```python
from build123d import *

# Parameters (mm, degrees)
BOSS_EXTRUDE1_DEPTH = 11.938
CUT_EXTRUDE1_DEPTH  = 11.43
SKETCH3_W           = 27.94
SKETCH3_H           = 25.845942769
CUT_EXTRUDE2_DEPTH  = 10.668
SKETCH4_R           = 1.905
CUT_EXTRUDE3_DEPTH  = 8.636
SKETCH5_R           = 1.143
CUT_EXTRUDE4_DEPTH  = 21.59
CUT_EXTRUDE5_DEPTH  = 2.54


with BuildPart() as part:
    # Sketch1 → Boss-Extrude1 (new body)
    with BuildSketch(Plane.XY):
        with BuildLine():
            Line((-4.737825132, -30.035944056), (-14.890307558, -23.641538462))
            ThreePointArc((-14.890307558, -23.641538462), (-27.242520167, -6.203925768), (-23.658870968, 14.862752926))
            ThreePointArc((-23.658870968, 14.862752926), (-20.55370118, 20.591203739), (-18.20732863, 26.67))
            Line((-18.20732863, 26.67), (18.20732863, 26.67))
            ThreePointArc((18.20732863, 26.67), (20.55370118, 20.591203739), (23.658870968, 14.862752926))
            ThreePointArc((23.658870968, 14.862752926), (27.242520167, -6.203925768), (14.890307558, -23.641538462))
            Line((14.890307558, -23.641538462), (4.737825132, -30.035944056))
            ThreePointArc((4.737825132, -30.035944056), (0, -31.403636364), (-4.737825132, -30.035944056))
        make_face()
    extrude(amount=BOSS_EXTRUDE1_DEPTH)

    # Sketch2 → Cut-Extrude1 (cut)
    with BuildSketch(Plane(origin=(0, 0, 0), x_dir=(-1, 0, 0), z_dir=(0, 0, -1))):
        with BuildLine():
            Line((-11.733590414, 23.241), (11.733590414, 23.241))
            ThreePointArc((11.733590414, 23.241), (0, -26.035), (-11.733590414, 23.241))
        make_face()
    extrude(amount=-CUT_EXTRUDE1_DEPTH, mode=Mode.SUBTRACT)

    # Sketch3 → Cut-Extrude2 (cut)
    with BuildSketch(Plane(origin=(0, 0, 0), x_dir=(-1, 0, 0), z_dir=(0, 0, -1))):
        with Locations((0, 24.280777857)):
            Rectangle(SKETCH3_W, SKETCH3_H)
    extrude(amount=-CUT_EXTRUDE2_DEPTH, mode=Mode.SUBTRACT)

    # Sketch4 → Cut-Extrude3 (cut)
    with BuildSketch(Plane.XY.offset(11.938)):
        with Locations((0, -28.575)):
            Circle(SKETCH4_R)
        with Locations((-16.764, 23.241)):
            Circle(SKETCH4_R)
        with Locations((16.764, 23.241)):
            Circle(SKETCH4_R)
    extrude(amount=-CUT_EXTRUDE3_DEPTH, mode=Mode.SUBTRACT)

    # Sketch5 → Cut-Extrude4 (cut)
    with BuildSketch(Plane.XY.offset(3.302)):
        with Locations((-16.764, 23.241)):
            Circle(SKETCH5_R)
        with Locations((16.764, 23.241)):
            Circle(SKETCH5_R)
        with Locations((0, -28.575)):
            Circle(SKETCH5_R)
    extrude(amount=-CUT_EXTRUDE4_DEPTH, mode=Mode.SUBTRACT)

    # Sketch6 → Cut-Extrude5 (cut)
    with BuildSketch(Plane(origin=(0, 0, 0), x_dir=(-1, 0, 0), z_dir=(0, 0, -1))):
        with BuildLine():
            Line((-23.658870968, 14.862752926), (-4.737825132, -30.035944056))
            ThreePointArc((-4.737825132, -30.035944056), (0, -31.403636364), (4.737825132, -30.035944056))
            Line((4.737825132, -30.035944056), (23.658870968, 14.862752926))
            ThreePointArc((23.658870968, 14.862752926), (20.55370118, 20.591203739), (18.20732863, 26.67))
            Line((18.20732863, 26.67), (-18.20732863, 26.67))
            ThreePointArc((-18.20732863, 26.67), (-20.55370118, 20.591203739), (-23.658870968, 14.862752926))
        make_face()
    extrude(amount=-CUT_EXTRUDE5_DEPTH, mode=Mode.SUBTRACT)


solid = part.part
```
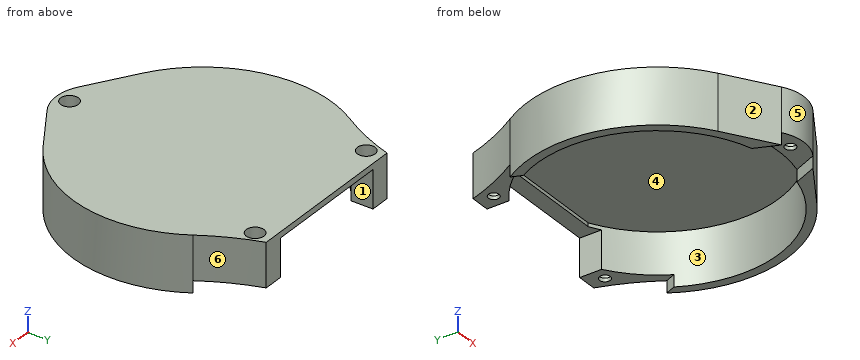
Geometry check sheet. Reference: the model listing, model coordinates, mm. Face numbers are marked on the shaded views. A direction names the side the tool comes from. Coordinates: 2 decimals unless noted, no trailing zeros. Write each loop counter-clockwise with the first axis right and the second up, starting at its lowest first coordinate (ties: lowest second). Pieces come first, ordered by that corner, then holes. Notation, with made-up numbers: M 10.25,9 L 56.25,9 A23 cw 56.25,40 Z; hole C 23,87.25 d9. An arc over 180 degrees is marked long. Answer as a JSON object with one key per item and string values.
1. Section check C-C, the plane y = 0. Enter the section's corners in (x, z) (3 decimals).
Answers below:
{"outline": "M -27.94,0 L -26.035,0 L -26.035,11.43 L 26.035,11.43 L 26.035,0 L 27.94,0 L 27.94,11.938 L -27.94,11.938 Z"}
2. Section check A-A, the plane z = 1.25. Enter the section's corners in (x, y) (3 decimals).
Answers below:
{"outline": "M -23.659,14.863 A27.94 ccw -14.89,-23.642 L -4.738,-30.036 L -6.805,-25.13 A26.035 cw -22.739,12.679 Z; M 4.738,-30.036 L 14.89,-23.642 A27.94 ccw 23.659,14.863 L 22.739,12.679 A26.035 cw 6.805,-25.13 Z"}
3. Section check B-B, the plane x = 0. Enter the section's corners in (y, z) (3 decimals).
Answers below:
{"outline": "M -31.404,2.54 L -29.718,2.54 L -29.718,3.302 L -30.48,3.302 L -30.48,11.938 L -31.404,11.938 Z; M -27.432,2.54 L -26.035,2.54 L -26.035,11.43 L 23.241,11.43 L 23.241,10.668 L 26.67,10.668 L 26.67,11.938 L -26.67,11.938 L -26.67,3.302 L -27.432,3.302 Z"}
4. Draft check along Y on the marked faces 3, 4, 5 and 6. Enter one of: released by +Y, released by -Y, zero draft, split by the parting line, or undercut.
Answers below:
{"face 3": "undercut", "face 4": "undercut", "face 5": "released by -Y", "face 6": "released by +Y"}
5. Scan lines: L1, parallel to X at y = 0, z = 4.25 (3 decimals); L2, parallel to Y at x = 17, z = 7; L3, parallel to Z at x = 4, y = 11. Record each from-to range of solid material in increasing order.
Answers below:
{"L1": "x = -27.94 to -26.035, 26.035 to 27.94", "L2": "y = -22.17 to -19.72, 19.72 to 21.35, 25.13 to 26.67", "L3": "z = 11.43 to 11.94"}
6. Go/stop test with flat-tipped pins: pin 1 Ø4 at (y, z) = (24, 6) entering from +X; pin 2 Ø5 at (x, y) = (5, 25) entering from -Z; pin 3 Ø7 at (x, y) = (-2.5, -27) entering from -Z; pin 4 Ø1.9 at (x, y) = (0, -28) entering from +Z. Record where each tip stops, or that it passes through.
Answers below:
{"pin 1": "stops at x = 19.93", "pin 2": "stops at z = 10.67", "pin 3": "stops at z = 0", "pin 4": "stops at z = 3.3"}
7. Tool access check on the marked faces 1 and 2. Record the directions out of +Z, -Z, +X, -X, +Y, -Y that give a thin tool (end or side, any length) a straight path to the whole face; none if there is none.
Answers below:
{"face 1": "-Z, +Y", "face 2": "+Z, -Z, -X, -Y"}
8. Section check D-D, the plane x = 13. Enter the section's corners in (y, z), plus the area to 3 significant figures.
Answers below:
{"outline": "M -24.83,0 L -22.56,0 L -22.56,11.43 L 22.56,11.43 L 22.56,10.67 L 26.67,10.67 L 26.67,11.94 L -24.83,11.94 Z", "area": "55.3 mm²"}
